```python
from build123d import *

# Parameters (mm, degrees)
F0_W     = 9.5
F0_H     = 42
F1_DEPTH = 19
F2_DEPTH = 456
F3_DEPTH = 23


with BuildPart() as f1:
    # F0 (on Front) → F1 (new body)
    with BuildSketch(Plane.XZ):
        Polygon((431, -229), (21, -229), (9.5, -229), (9.5, -271), (431, -271), align=None)
        Polygon((9.5, -229), (21, -229), (21, 229), (0, 229), (-21, 229), (-21, -229), (-9.5, -229), (0, -229), align=None)
        with Locations((4.75, -250)):
            Rectangle(F0_W, F0_H)
        Polygon((0, 229), (21, 229), (450, 229), (450, 248), (0, 248), align=None)
        with Locations((-4.75, -250)):
            Rectangle(F0_W, F0_H)
        Polygon((-21, 229), (0, 229), (0, 248), (-450, 248), (-450, 229), align=None)
        Polygon((-9.5, -271), (-9.5, -229), (-21, -229), (-431, -229), (-431, -271), align=None)
    extrude(amount=F1_DEPTH)

    # F0 (on Front) → F2 (join)
    with BuildSketch(Plane.XZ):
        with Locations((-4.75, -250)):
            Rectangle(F0_W, F0_H)
        with Locations((4.75, -250)):
            Rectangle(F0_W, F0_H)
    extrude(amount=-F2_DEPTH)

    # F0 (on Front) → F3 (join)
    with BuildSketch(Plane.XZ):
        Polygon((0, 229), (21, 229), (450, 229), (450, 248), (0, 248), align=None)
        Polygon((-21, 229), (0, 229), (0, 248), (-450, 248), (-450, 229), align=None)
    extrude(amount=-F3_DEPTH)


solid = f1.part
```
The listing builds one solid part. Answer for the finished solid, in the listing's coordinates (mm). A direction names the side the tool comes from. Give positions to 0.01 mm unless a question says otherwise; leave off trailing zeros. Order: outer loops, then holes, each group sorted by start corner. A loop starts at its lowest first (then second) coordinate and runs counter-clockwise, first axis right, second up.
Item 1: Find the intervals of material crossed by probe 1 along Z at (x, y) = (-370, 3), in increasing order.
From the geometry:
probe 1: z = 229 to 248
Item 2: The part is cut by section B-B, the plane y = 104. Give the vertices of the cut face in (x, z), and give its area (3 significant figures).
From the geometry:
outline: (-9.5, -271) - (9.5, -271) - (9.5, -229) - (-9.5, -229) - close
area: 798 mm2
Item 3: Which of the six approach directions +Z, -Z, +X, -X, +Y, -Y give full straight-line access (tool end or side, diameter ignored) to faces 1 (the face through (-431, -9, -250)), 2 (the face through (21, -9, -3)), 3 (the face through (431, -9, -250)), 4 (the face through (-223, -9, -229))?
From the geometry:
face 1: -Z, -X, +Y, -Y
face 2: +X, +Y, -Y
face 3: -Z, +X, +Y, -Y
face 4: -X, +Y, -Y
Item 4: Given pin 1 Ø21 at (y, z) = (-9, -96.5) entering from -X; pin 2 Ø21 at (y, z) = (248, -254.5) entering from -X; pin 3 Ø15 at (x, z) = (-102.5, 241) entering from +Y; pin 4 Ø21 at (x, y) = (-115.5, 10) entering from -Z, each flat-ended and moving along its own axis, determine where each tip first touches the part or whether it passes through.
From the geometry:
pin 1: stops at x = -21
pin 2: stops at x = -9.5
pin 3: stops at y = 23
pin 4: stops at z = -271
Item 5: The part is cut by section C-C, the plane z = -65. Give the vertices of the cut face in (x, y).
From the geometry:
outline: (-21, -19) - (21, -19) - (21, 0) - (-21, 0) - close
Item 6: For a pull along Z with two mould halves and no side action, classify faces 5 (the face through (6, 2, 248)), 6 (the face through (-21, -9, 3)), 7 (the face through (-6, 2, 229)), 8 (the face through (-6, 23, 239)) as pulls with the +Z half, pulls with the -Z half, needs draft (parallel to the pull), parting line crosses it, or undercut.
From the geometry:
face 5: pulls with the +Z half
face 6: undercut
face 7: undercut
face 8: needs draft
Item 7: The part is cut by section A-A, the plane x = -344.5. Give the vertices of the cut face in (y, z).
From the geometry:
outline: (-19, -271) - (0, -271) - (0, -229) - (-19, -229) - close; (-19, 229) - (23, 229) - (23, 248) - (-19, 248) - close
